from build123d import *

# Parameters (mm, degrees)
SKETCH1_W           = 1150
SKETCH1_H           = 440
SKETCH1_W_2         = 1070
SKETCH1_H_2         = 350
BOSS_EXTRUDE1_DEPTH = 6
SKETCH3_R           = 2.5
CUT_EXTRUDE2_DEPTH  = 618.483603021
SKETCH2_W           = 1112
SKETCH2_H           = 402
SKETCH2_W_2         = 1070
SKETCH2_H_2         = 350
CUT_EXTRUDE1_DEPTH  = 3
BOSS_EXTRUDE2_DEPTH = 6
SKETCH5_W           = 6
SKETCH5_H           = 69
BOSS_EXTRUDE3_DEPTH = 26
CUT_EXTRUDE3_DEPTH  = 26
FILLET1_R           = 5


with BuildPart() as part:
    # Sketch1 → Boss-Extrude1 (new body)
    with BuildSketch(Plane.XY):
        with Locations((0, 5)):
            Rectangle(SKETCH1_W, SKETCH1_H)
        Rectangle(SKETCH1_W_2, SKETCH1_H_2, mode=Mode.SUBTRACT)
    extrude(amount=BOSS_EXTRUDE1_DEPTH)

    # Sketch3 → Cut-Extrude2 (cut, through all)
    with BuildSketch(Plane(origin=(0, 0, 0), x_dir=(-1, 0, 0), z_dir=(0, 0, -1))):
        with Locations((-565.5, 215.5)):
            Circle(SKETCH3_R)
        with Locations((565.5, 215.5)):
            Circle(SKETCH3_R)
        with Locations((565.5, -205.5)):
            Circle(SKETCH3_R)
        with Locations((-565.5, -205.5)):
            Circle(SKETCH3_R)
    extrude(amount=-CUT_EXTRUDE2_DEPTH, mode=Mode.SUBTRACT)

    # Sketch2 → Cut-Extrude1 (cut)
    with BuildSketch(Plane(origin=(0, 0, 0), x_dir=(-1, 0, 0), z_dir=(0, 0, -1))):
        with Locations((0, 5)):
            Rectangle(SKETCH2_W, SKETCH2_H)
        Rectangle(SKETCH2_W_2, SKETCH2_H_2, mode=Mode.SUBTRACT)
    extrude(amount=-CUT_EXTRUDE1_DEPTH, mode=Mode.SUBTRACT)

    # Sketch4 → Boss-Extrude2 (add)
    with BuildSketch(Plane.XY.offset(6)):
        Polygon((0, 175), (0, 103), (20, 103), (70, 175), align=None)
    extrude(amount=-BOSS_EXTRUDE2_DEPTH)

    # Sketch5 → Boss-Extrude3 (add)
    with BuildSketch(Plane.XY.offset(6)):
        with Locations((-3, 137.5)):
            Rectangle(SKETCH5_W, SKETCH5_H)
    extrude(amount=-BOSS_EXTRUDE3_DEPTH)

    # Sketch6 → Cut-Extrude3 (cut)
    with BuildSketch(Plane(origin=(0, 0, 0), x_dir=(0, 0, -1), z_dir=(1, 0, 0))):
        with BuildLine():
            Line((13, 162), (13, 113))
            ThreePointArc((13, 113), (10, 110), (7, 113))
            Line((7, 113), (7, 162))
            ThreePointArc((7, 162), (10, 165), (13, 162))
        make_face()
    extrude(amount=-CUT_EXTRUDE3_DEPTH, mode=Mode.SUBTRACT)

    # Fillet1
    fillet1_edges = [part.edges().sort_by_distance(p)[0] for p in [
        (20, 103, 3),
        (-3, 103, -20),
        (-3, 172, -20),
        (-6, 137.5, 6),
    ]]
    fillet(fillet1_edges, radius=FILLET1_R)


solid = part.part
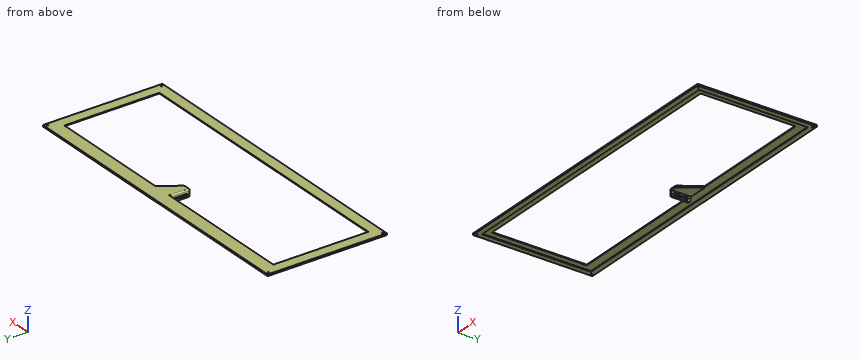
CAD build for the part. Positions are in the model's coordinates, mm. Round coordinates to 2 decimals unless told otherwise and drop trailing zeros. Order: outer loops, then holes, each group sorted by start corner. A loop starts at its lowest first (then second) coordinate and runs counter-clockwise, first axis right, second up. Notation, with made-up numbers: (88.25, 89) - (94.25, 89) arc R18 ccw to (94.25, 120) - close; hole circle Ø1 at (-20.5, 45.25). An arc over 180 degrees is marked (long way). Return JSON: item names as keys, results as strings.
(1) Cut at A-A (y = 11.5). Give the cut face in (x, z), then the cut area to 3 significant figures.
Answer key:
{"outline": "(-575, 0) - (-556, 0) - (-556, 3) - (-535, 3) - (-535, 6) - (-575, 6) - close; (535, 3) - (556, 3) - (556, 0) - (575, 0) - (575, 6) - (535, 6) - close", "area": "354 mm^2"}
(2) Cut at C-C (x = 59). Give the cut face in (y, z).
Answer key:
{"outline": "(-215, 0) - (-196, 0) - (-196, 3) - (-175, 3) - (-175, 6) - (-215, 6) - close; (159.16, 0) - (175, 0) - (175, 3) - (206, 3) - (206, 0) - (225, 0) - (225, 6) - (159.16, 6) - close"}
(3) Wall check: probe 1 along Y at (x, z) = (565.5, 4.2); probe 2 along X at (y, z) = (215.5, 4.1); probe 3 along X at (y, z) = (-88, 3.5). Give the ranges that are in metal, low to high. Write a range as from..to.
Answer key:
{"probe 1": "y = -215..-208, -203..213, 218..225", "probe 2": "x = -575..-568, -563..563, 568..575", "probe 3": "x = -575..-535, 535..575"}
(4) Pin check, flat tips, straight feed: pin 1 Ø10 at (y, z) = (137, -12.5) entering from +X; pin 2 Ø6.5 at (y, z) = (146.5, -4.5) entering from -X; pin 3 Ø10 at (x, z) = (-1, -7.5) entering from +Y. Stop position of each tip, or through.
Answer key:
{"pin 1": "stops at x = 0", "pin 2": "stops at x = -6", "pin 3": "stops at y = 172"}
(5) Cut at B-B (x = 366). Give the cut face in (y, z).
Answer key:
{"outline": "(-215, 0) - (-196, 0) - (-196, 3) - (-175, 3) - (-175, 6) - (-215, 6) - close; (175, 3) - (206, 3) - (206, 0) - (225, 0) - (225, 6) - (175, 6) - close"}
